Part print with two shaded views. Sizes in mm from the minimum x, y, z corner. Give positions to 0.01 mm unless a question says otherwise; leave off trailing zeros. Write each loop counter-clockwise with the first axis right and the second up, starting at its lowest first coordinate (ties: lowest second). Pieces come first, ordered by that corner, then holes.
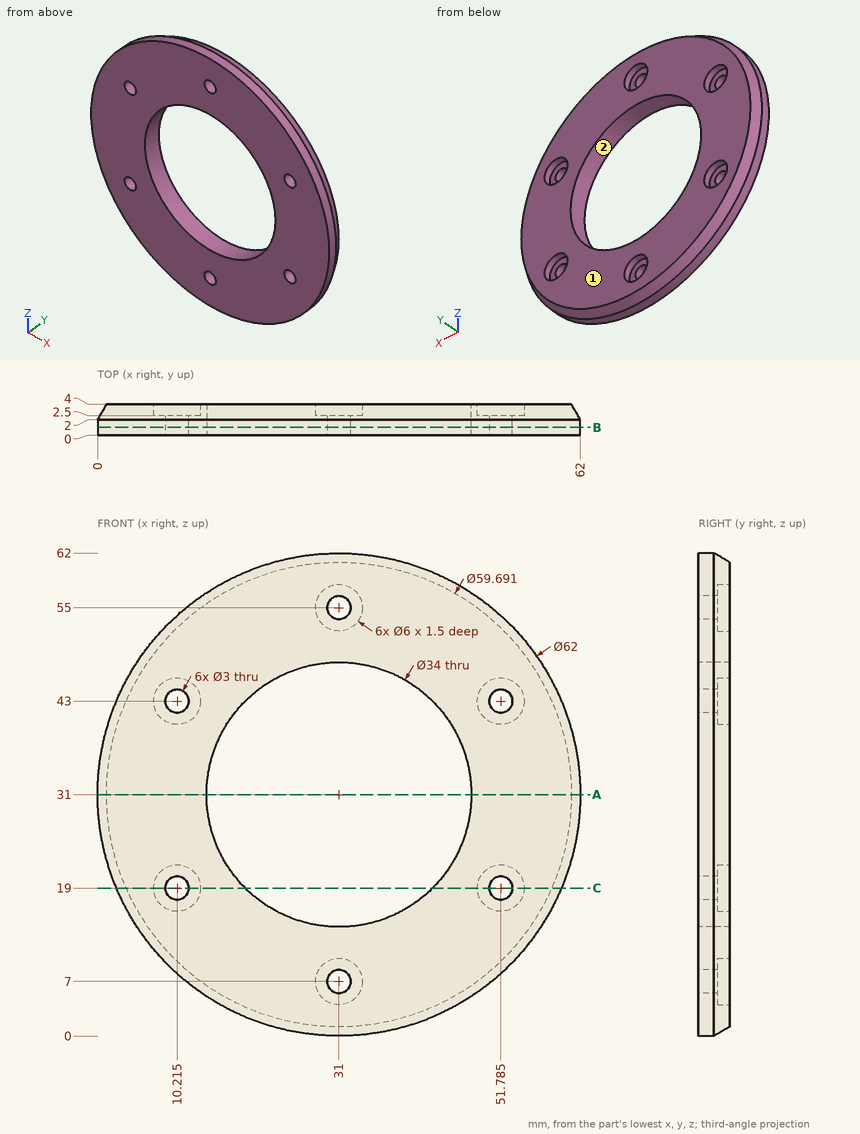
1) Saw through at C-C, the plane z = 19. Count the separate pieces of the cut face and the enclosed holes in it.
Answers follow:
separate pieces: 4
enclosed holes: 0
2) Saw through at A-A, the plane z = 31. Write the cut outline in (x, y) (1 decimal), then the cut area to 3 significant figures.
Answers follow:
outline: (0, 0) - (14, 0) - (14, 4) - (1.2, 4) - (0, 2) - close; (48, 0) - (62, 0) - (62, 2) - (60.8, 4) - (48, 4) - close
area: 110 mm2
3) Saw through at B-B, the plane y = 1. Write the cut outline in (x, z) (1 decimal), then the cut area to 3 significant figures.
Answers follow:
outline: circle Ø62 at (31, 31); hole circle Ø3 at (10.2, 19); hole circle Ø3 at (10.2, 43); hole circle Ø34 at (31, 31); hole circle Ø3 at (31, 7); hole circle Ø3 at (31, 55); hole circle Ø3 at (51.8, 19); hole circle Ø3 at (51.8, 43)
area: 2,070 mm2
4) Two-plate mould, pull along Z, no slides. Class the marked faces 1 and 2: +Z half, -Z half, draft (parallel to the pull), parting line (faces both ways), or undercut.
Answers follow:
face 1: draft
face 2: undercut
5) Pin check, flat tips, straight feed: pin 1 Ø5.5 at (x, z) = (31, 7) entering from +Y; pin 2 Ø5 at (x, z) = (10.5, 20) entering from +Y; pin 3 Ø2 at (y, z) = (2.5, 22.5) entering from -X (1 decimal); pin 4 Ø1.5 at (y, z) = (0.5, 42.5) entering from +X. Stop position of each tip, or through.
Answers follow:
pin 1: stops at y = 2.5
pin 2: stops at y = 4
pin 3: stops at x = 1
pin 4: stops at x = 60.08
6) Wall check: L1, parallel to Z at x = 52, y = 2.25 (1 decimal); L2, parallel to X at y = 0.25, z = 18.5; L3, parallel to X at y = 2.55, z = 19 (1 decimal). Give the ranges that are in metal, low to high.
Answers follow:
L1: z = 8.4 to 17.5, 20.5 to 41.5, 44.5 to 53.6
L2: x = 2.63 to 8.8, 11.63 to 19.48, 42.52 to 50.37, 53.2 to 59.37
L3: x = 2.8 to 7.2, 13.2 to 19, 43 to 48.8, 54.8 to 59.2
